from build123d import *

# Parameters (mm, degrees)
EXTRUDE_1_DEPTH     = 27
SKETCH_2_W          = 10
SKETCH_2_H          = 9
CUT_EXTRUDE_1_DEPTH = 5


with BuildPart() as part:
    # 草图1 → 凸台-拉伸1 (new body)
    with BuildSketch(Plane.XY):
        Polygon((0, 0), (10, 0), (10, -32.6), (-5, -32.6), (-5, -20), (0, -20), (0, -13), (-5, -13), (-5, -7), (0, -7), align=None)
    extrude(amount=EXTRUDE_1_DEPTH)

    # 草图2 → 切除-拉伸1 (cut)
    with BuildSketch(Plane(origin=(0, 0, 0), x_dir=(1, 0, 0), z_dir=(0, 1, 0))):
        with Locations((5, -13.5)):
            Rectangle(SKETCH_2_W, SKETCH_2_H)
    extrude(amount=-CUT_EXTRUDE_1_DEPTH, mode=Mode.SUBTRACT)


solid = part.part
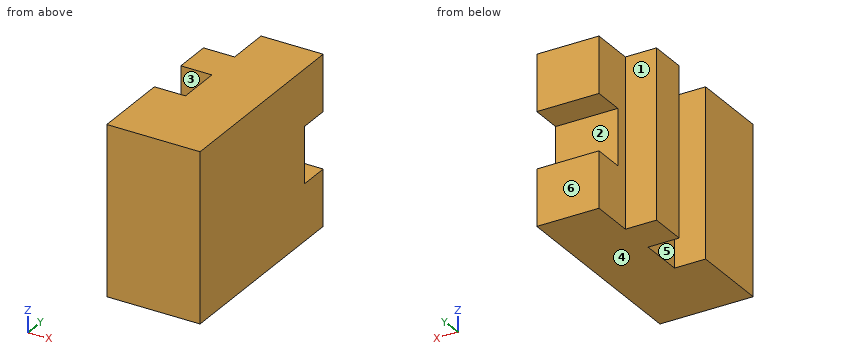
Input: part model. Units: mm. Frame: model coordinates. Face numbers are marked on the shaded views. A direction names the side the tool comes from. Give positions to 0.01 mm unless a question says otherwise; leave off trailing zeros. Write each loop counter-clockwise with the first axis right and the second up, starting at its lowest first coordinate (ties: lowest second). Pieces come first, ordered by that corner, then holes. Notation, with made-up numbers: M -38,-29 L -25,-29 A16 ccw -25,-15 Z; hole C 47,-7 d4. An arc over 180 degrees is marked long. Use one line per item in the form item = value.
1. Cut plane D-D on x = 0.5. Return loops of the section in (y, z).
Outcome:
outline = M -32.6,0 L 0,0 L 0,9 L -5,9 L -5,18 L 0,18 L 0,27 L -32.6,27 Z
2. Ray query, L1, parallel to Y at x = -3.25, z = 10.25; L2, parallel to Y at x = 0.25, z = 12.25; L3, parallel to X at y = -5, z = 7.75. Return the intervals inside material, ascending.
Outcome:
L1 = -32.6 to -20, -13 to -7
L2 = -32.6 to -5
L3 = 0 to 10
3. Cut plane C-C on z = 25. Return loops of the section in (x, y).
Outcome:
outline = M -5,-32.6 L 10,-32.6 L 10,0 L 0,0 L 0,-7 L -5,-7 L -5,-13 L 0,-13 L 0,-20 L -5,-20 Z
4. First-contact query: P1, Ø7.5, axis at y = -3.5, z = 11, coming from the -X side; P2, Ø4.5, axis at x = 6.5, z = 12.5, coming from the +Y side; P3, Ø5.5, axis at y = -16.5, z = 8, coming from the -X side; P4, Ø1.5, axis at x = -3.5, z = 8, coming from the +Y side. Flat tips, straight axial feed; report the tip coordinate or a pass-through.
Outcome:
P1 = -5
P2 = -5
P3 = 0
P4 = -7
5. Cut plane B-B on y = -2. Return loops of the section in (x, z), and give its area (3 significant figures).
Outcome:
outline = M 0,0 L 10,0 L 10,9 L 0,9 Z; M 0,18 L 10,18 L 10,27 L 0,27 Z
area = 180 mm²
6. Cut plane A-A on x = -2.25. Return loops of the section in (y, z), and give its area (3 significant figures).
Outcome:
outline = M -32.6,0 L -20,0 L -20,27 L -32.6,27 Z; M -13,0 L -7,0 L -7,27 L -13,27 Z
area = 502 mm²
7. Mould query, pull axis Y, two halves, no side actions, for the marked faces 4, 5 and 6. Classes: released by +Y, released by -Y, zero draft, split by the parting line, or undercut.
Outcome:
face_4 = zero draft
face_5 = undercut
face_6 = released by +Y
8. Reachability of the marked faces 1, 2 and 3 from +Z, -Z, +X, -X, +Y, -Y: full face, straight path, thin tool, end or side. Return the list, or none.
Outcome:
face_1 = +Z, -Z, -X, +Y
face_2 = +X, -X, +Y
face_3 = +Z, -Z, -X
